Source: three-view drawing plus pictorial views. Frame: mm from the lowest corner of the part. Give positions to 0.01 mm unless a question says otherwise; leave off trailing zeros. Order: outer loops, then holes, each group sorted by start corner. A loop starts at its lowest first (then second) coordinate and runs counter-clockwise, first axis right, second up. Notation, with made-up numbers: (-16.5, 80.25) -> (33.5, 80.25) arc R12 cw to (33.5, 97.25) -> close; hole circle Ø8 at (42, 14.5). An arc over 180 degrees is marked (long way). Answer in a Markdown table with one row per item.
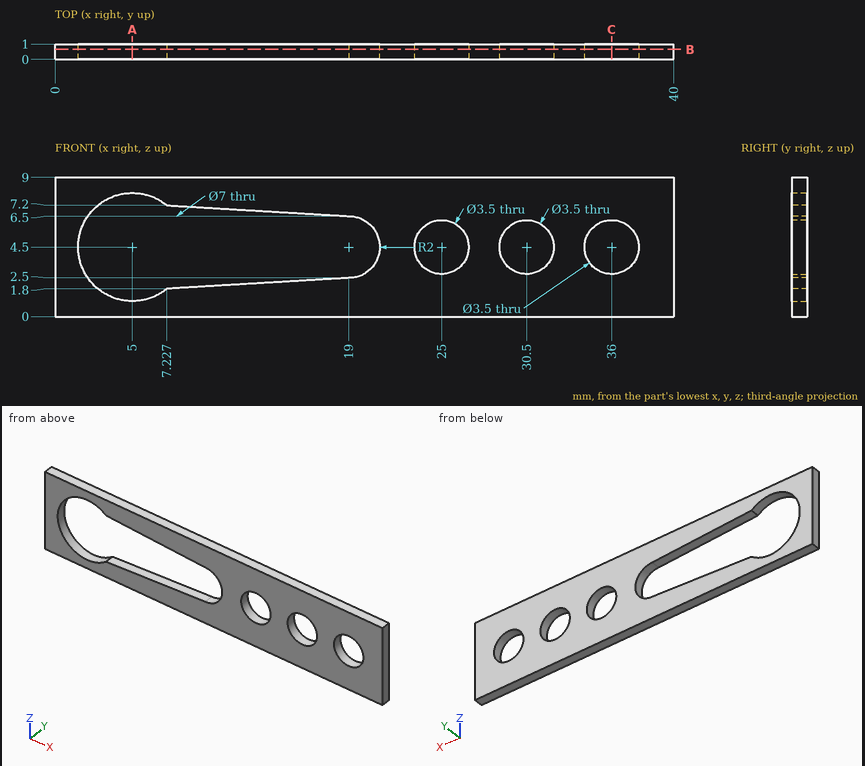
(1) Section query C-C (x = 36). Return the cut outline in (y, z), plus the area to 3 significant figures.
A:
| item | result |
|---|---|
| outline | (0, 0) -> (1, 0) -> (1, 2.75) -> (0, 2.75) -> close; (0, 6.25) -> (1, 6.25) -> (1, 9) -> (0, 9) -> close |
| area | 5.50 mm^2 |
(2) Section query B-B (y = 0.65). Return the cut outline in (x, z), plus the area to 3 significant figures.
A:
| item | result |
|---|---|
| outline | (0, 0) -> (40, 0) -> (40, 9) -> (0, 9) -> close; hole (7.23, 1.8) -> (19, 2.5) arc R2 ccw to (19, 6.5) -> (7.23, 7.2) arc R3.5 ccw (long way) to start; hole circle Ø3.5 at (25, 4.5); hole circle Ø3.5 at (30.5, 4.5); hole circle Ø3.5 at (36, 4.5) |
| area | 236 mm^2 |
(3) First-contact query: pin 1 Ø2 at (x, z) = (30.5, 4.5) entering from +Y. Flat tip, straight axial feed; report the tip coordinate or a pass-through.
A:
| item | result |
|---|---|
| pin 1 | passes through |
(4) Section query A-A (x = 5). Return the cut outline in (y, z), plus the area to 3 significant figures.
A:
| item | result |
|---|---|
| outline | (0, 0) -> (1, 0) -> (1, 1) -> (0, 1) -> close; (0, 8) -> (1, 8) -> (1, 9) -> (0, 9) -> close |
| area | 2.00 mm^2 |
(5) Ray query, probe 1 along X at (y, z) = (0.65, 4.5); probe 2 along Z at (x, y) = (36, 0.55); probe 3 along X at (y, z) = (0.65, 6). Return the intervals inside material, ascending.
A:
| item | result |
|---|---|
| probe 1 | x = 0 to 1.5, 21 to 23.25, 26.75 to 28.75, 32.25 to 34.25, 37.75 to 40 |
| probe 2 | z = 0 to 2.75, 6.25 to 9 |
| probe 3 | x = 0 to 1.84, 20.32 to 24.1, 25.9 to 29.6, 31.4 to 35.1, 36.9 to 40 |
